```python
from build123d import *

# Parameters (mm, degrees)
RESSALTO_EXTRUS_O1_DEPTH = 10
ESBO_O2_R                = 3.25
CORTE_EXTRUS_O1_DEPTH    = 10
ESBO_O3_R                = 1.5
CORTE_EXTRUS_O2_DEPTH    = 10
CORTE_EXTRUS_O3_START    = 10
ESBO_O4_R                = 3.25
CORTE_EXTRUS_O3_DEPTH    = 10
ESBO_O5_W                = 16
ESBO_O5_H                = 40
ESBO_O5_R                = 1.75
RESSALTO_EXTRUS_O2_DEPTH = 4
CHANFRO1_SIZE            = 5
CHANFRO2_SIZE            = 5
CHANFRO3_SIZE            = 1


with BuildPart() as part:
    # Esboço1 → Ressalto-extrusão1 (new body)
    with BuildSketch(Plane.XY):
        with BuildLine():
            Line((0, 8.5), (8.5, 8.5))
            Line((8.5, 8.5), (8.5, 0))
            Line((8.5, 0), (8.5, -8.5))
            Line((8.5, -8.5), (0, -8.5))
            ThreePointArc((0, -8.5), (-4.626013402, -7.130918594), (-7.761817645, -3.464705882))
            Line((-7.761817645, -3.464705882), (-10.984889326, -3.464705686))
            Line((-10.984889326, -3.464705686), (-10.984889326, -0.964705686))
            Line((-10.984889326, -0.964705686), (-3.984889326, -0.964705686))
            ThreePointArc((-3.984889326, -0.964705686), (4.1, -1.01e-07), (-3.984889278, 0.964705882))
            Line((-3.984889278, 0.964705882), (-10.984889278, 0.964705882))
            Line((-10.984889278, 0.964705882), (-10.984889278, 3.464705882))
            Line((-10.984889278, 3.464705882), (-7.761817645, 3.464705882))
            ThreePointArc((-7.761817645, 3.464705882), (-4.626013402, 7.130918594), (0, 8.5))
        make_face()
    extrude(amount=RESSALTO_EXTRUS_O1_DEPTH)

    # Esboço2 → Corte-extrusão1 (cut)
    with BuildSketch(Plane(origin=(0, 3.464705882, 0), x_dir=(1, 0, 0), z_dir=(0, 1, 0))):
        with Locations((-9.261817645, -4.955566824)):
            Circle(ESBO_O2_R)
    extrude(amount=CORTE_EXTRUS_O1_DEPTH, mode=Mode.SUBTRACT)

    # Esboço3 → Corte-extrusão2 (cut)
    with BuildSketch(Plane(origin=(0, 3.464705882, 0), x_dir=(1, 0, 0), z_dir=(0, 1, 0))):
        with Locations(Location((-9.261817645, -4.955566824, 0), (0, 0, 180))):
            Circle(ESBO_O3_R)
    extrude(amount=-CORTE_EXTRUS_O2_DEPTH, mode=Mode.SUBTRACT)

    # Esboço4 → Corte-extrusão3 (cut)
    with BuildSketch(Plane(origin=(-2.11e-07, -3.464706354, 0), x_dir=(-0.9999999999999982, 6.08161782252128e-08, 0), z_dir=(-6.081617822521279e-08, -0.9999999999999981, 0)).offset(CORTE_EXTRUS_O3_START)):
        with Locations((9.261817434, -4.955566824)):
            Circle(ESBO_O4_R)
    extrude(amount=-CORTE_EXTRUS_O3_DEPTH, mode=Mode.SUBTRACT)

    # Esboço5 → Ressalto-extrusão2 (add)
    with BuildSketch(Plane(origin=(6, 0, 0), x_dir=(0, 0, -1), z_dir=(1, 0, 0))):
        with Locations((-2, 7)):
            Rectangle(ESBO_O5_W, ESBO_O5_H)
        with Locations((3.5, 9.5)):
            Circle(ESBO_O5_R, mode=Mode.SUBTRACT)
        with Locations((3.5, -9.5)):
            Circle(ESBO_O5_R, mode=Mode.SUBTRACT)
    extrude(amount=RESSALTO_EXTRUS_O2_DEPTH)

    # Chanfro1
    chanfro1_edges = [part.edges().sort_by_distance(p)[0] for p in [
        (6, 8.5, 5),
    ]]
    chamfer(chanfro1_edges, length=CHANFRO1_SIZE)

    # Chanfro2
    # the kernel refuses this chamfer: 5 mm, written as the material it adds along each edge
    with BuildSketch(Plane(origin=(6, -8.5, 10), x_dir=(-0.9996219169112968, 0.027495876610586317, 0), z_dir=(0, 0, -1))) as chanfro2_piece_1_section:
        Polygon((CHANFRO2_SIZE * 0.999621916911, -CHANFRO2_SIZE * 0.0274958766106), (-CHANFRO2_SIZE * 0.0274958766106, -CHANFRO2_SIZE * 0.999621916911), (0, 0), align=None)
    chanfro2_piece_1 = extrude(amount=10, mode=Mode.PRIVATE)
    chanfro2_piece_1 = split(chanfro2_piece_1, bisect_by=Plane(origin=(4.320496265, -13, 5), z_dir=(0, 1, 0)), keep=Keep.TOP, mode=Mode.PRIVATE)
    add(chanfro2_piece_1)

    # Chanfro3
    # the kernel refuses this chamfer: 1 mm, written as the material it takes off along each edge
    with BuildSketch(Plane(origin=(6, -13, -8.571682988), x_dir=(-0.02749587661058651, 0.9996219169112968, 0), z_dir=(0, 0, 1))) as chanfro3_piece_1:
        Polygon((CHANFRO3_SIZE * 0.999621916911, -CHANFRO3_SIZE * 0.0274958766106), (-CHANFRO3_SIZE * 0.0274958766106, -CHANFRO3_SIZE * 0.999621916911), (0, 0), align=None)
    extrude(amount=8.571682988, mode=Mode.SUBTRACT)
    with BuildSketch(Plane(origin=(6, 10.928317012, 10), x_dir=(-0.02749587661058651, 0, -0.9996219169112968), z_dir=(0, 1, 0))) as chanfro3_piece_2_section:
        Polygon((CHANFRO3_SIZE * 0.999621916911, -CHANFRO3_SIZE * 0.0274958766106), (-CHANFRO3_SIZE * 0.0274958766106, -CHANFRO3_SIZE * 0.999621916911), (0, 0), align=None)
    chanfro3_piece_2 = extrude(amount=18.643365976, mode=Mode.PRIVATE)
    chanfro3_piece_2 = split(chanfro3_piece_2, bisect_by=Plane(origin=(10.262240478, 17.762240478, 9.668049788), z_dir=(-0.7071067811865476, 0.7071067811865476, 0)), keep=Keep.TOP, mode=Mode.PRIVATE)
    add(chanfro3_piece_2, mode=Mode.SUBTRACT)
    with BuildSketch(Plane(origin=(6, 29.571682988, -6), x_dir=(-0.027495876610586487, 0, 0.9996219169112968), z_dir=(0, -1, 0))) as chanfro3_piece_3:
        Polygon((CHANFRO3_SIZE * 0.999621916911, -CHANFRO3_SIZE * 0.0274958766106), (-CHANFRO3_SIZE * 0.0274958766106, -CHANFRO3_SIZE * 0.999621916911), (0, 0), align=None)
    extrude(amount=45.143365976, mode=Mode.SUBTRACT)
    with BuildSketch(Plane(origin=(6, 27, 12.571682988), x_dir=(-0.02749587661058651, -0.9996219169112968, 0), z_dir=(0, 0, -1))) as chanfro3_piece_4:
        Polygon((CHANFRO3_SIZE * 0.999621916911, -CHANFRO3_SIZE * 0.0274958766106), (-CHANFRO3_SIZE * 0.0274958766106, -CHANFRO3_SIZE * 0.999621916911), (0, 0), align=None)
    extrude(amount=21.143365976, mode=Mode.SUBTRACT)


solid = part.part
```
Here's how the part is built. I have some questions about the finished solid (model axes, mm). A direction names the side the tool comes from. Give positions to 0.01 mm unless a question says otherwise; leave off trailing zeros. Loops run counter-clockwise (first coordinate to the right, second up) from the corner with the lowest first, then second, coordinate; pieces in that order, holes last. Notation, with made-up numbers: M 50,57 L 55,57 A23 ccw 55,92 Z; hole C -12.75,16 d2. An arc over 180 degrees is marked long. Return JSON: item names as keys, results as strings.
Item 1: Imagine slicing it at C-C on x = -1.5. List the corners of the cut face in (y, z) for me, then the cut area to 3 significant figures.
A:
{"outline": "M -8.37,0 L -3.82,0 L -3.82,10 L -8.37,10 Z; M 3.82,0 L 8.37,0 L 8.37,10 L 3.82,10 Z", "area": "91.0 mm^2"}
Item 2: Imagine slicing it at A-A on y = 9.5. List the corners of the cut face in (x, z) for me.
A:
{"outline": "M 2,0 L 6,0 L 6,-1.75 L 10,-1.75 L 10,10 L 2,10 Z; M 6.25,-5.25 L 7,-6 L 10,-6 L 10,-5.25 Z"}
Item 3: Please list where these lines run through material, in increasing order: line 1 (Y direction, x = 7.3, z = -3.5); line 2 (Y direction, x = 6.75, z = -3); line 3 (X direction, y = 2, z = 6).
A:
{"line 1": "y = -13 to -11.25, -7.75 to 7.75, 11.25 to 27", "line 2": "y = -12.75 to -11.18, -7.82 to 7.82, 11.18 to 26.75", "line 3": "x = -10.98 to -10.34, -8.19 to -3.58, 3.58 to 10"}
Item 4: Imagine slicing it at D-D on y = 2. List the corners of the cut face in (x, z) for me.
A:
{"outline": "M -10.98,0 L -3.58,0 L -3.58,10 L -10.98,10 Z; M 3.58,0 L 6,0 L 6,-5 L 7,-6 L 10,-6 L 10,10 L 3.58,10 Z; hole C -9.26,4.96 d3"}
Item 5: On a 3-axis mill with a long thin cutter (end or side, diameter ignored), from which of +Z, -Z, +X, -X, +Y, -Y can I reach the whole of each face in a straight line? I mean faces 1 (the cylindrical face through (-6.012, 4.436, 5.005)), 2 (the flat face through (0.5, -8.5, 4.9)), 3 (the flat face through (-7.5, -0.965, 4.9)), 4 (the cylindrical face through (-6.012, -4.472, 4.906)). Say none if no direction works.
A:
{"face 1": "-X, +Y", "face 2": "+Z, -Z, -X, -Y", "face 3": "+Z, -Z, -X", "face 4": "-X, -Y"}
Item 6: I'm going to push flat-ended pins straight in: pin 1 Ø5.5 at (x, z) = (-9, 2.5) entering from -Y; pin 2 Ø4 at (y, z) = (-9.5, -3.5) entering from +X; pin 3 Ø2.5 at (x, z) = (-10, 7.5) entering from -Y; pin 4 Ø12 at (x, y) = (-4, -4) entering from -Z. Where does each tip first touch, or does it pass through?
A:
{"pin 1": "stops at y = -5.76", "pin 2": "stops at x = 10", "pin 3": "stops at y = -3.46", "pin 4": "stops at z = 0"}
Item 7: Imagine slicing it at B-B on z = -3.5. List the corners of the cut face in (x, y) for me.
A:
{"outline": "M 6,-12 L 7,-13 L 10,-13 L 10,-11.25 L 6,-11.25 Z; M 6,-7.75 L 10,-7.75 L 10,7.75 L 6,7.75 Z; M 6,11.25 L 10,11.25 L 10,27 L 7,27 L 6,26 Z"}
Item 8: Thinking about a two-plate mould opening in Y: for faces 5 (the flat face through (3.2, -10.7, 5.1)), 6 (the cylindrical face through (4.097, -0.167, 4.93)), 7 (the flat face through (6.5, 20.2, 9.5)), which applies, released by +Y, released by -Y, zero draft, split by the parting line, or undercut?
A:
{"face 5": "released by -Y", "face 6": "undercut", "face 7": "zero draft"}
